Here's the drawing with two shaded views (mm, measured from the low corner). I have some questions. A direction names the side the tool comes from. Give positions to 0.01 mm unless a question says otherwise; leave off trailing zeros. Loops run counter-clockwise (first coordinate to the right, second up) from the corner with the lowest first, then second, coordinate; pieces in that order, holes last. Notation, with made-up numbers: (59, 32.5) - (85, 32.5) arc R8 cw to (85, 43.5) - close; hole circle Ø5 at (72, 58.25). An arc over 180 degrees is marked (long way). Use one line per item in the form item = value.
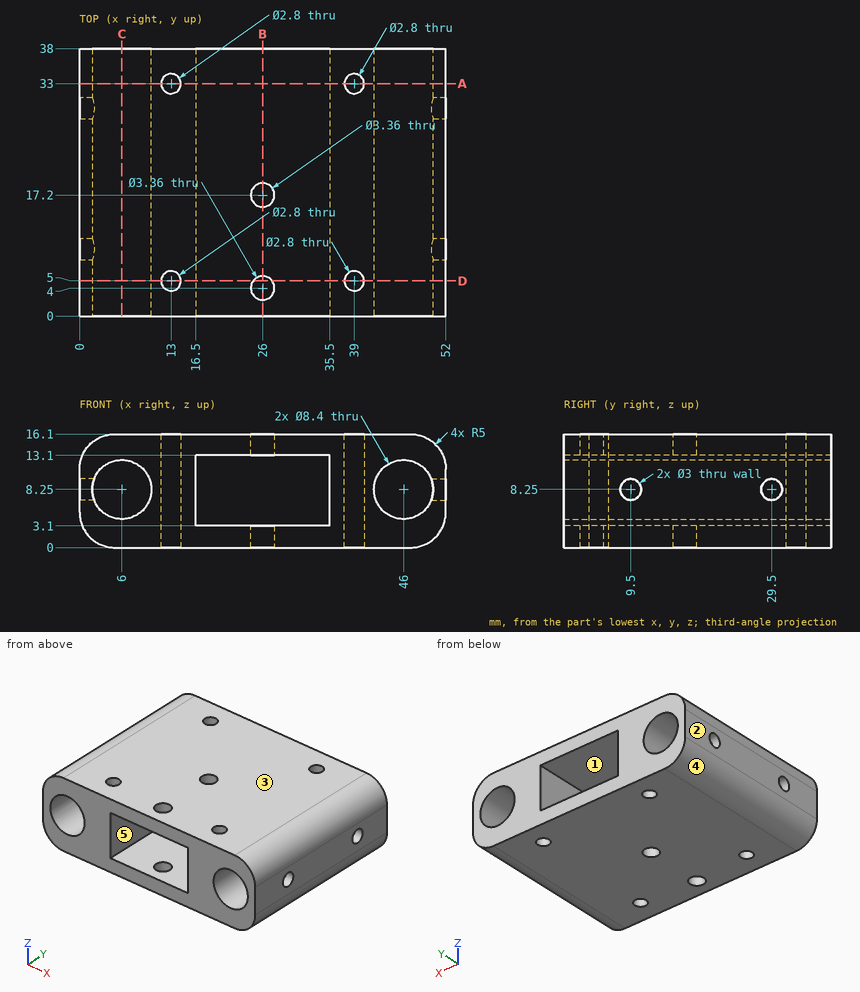
(1) For the marked faces 4 and 5, which set-ups out of +Z, -Z, +X, -X, +Y, -Y let a thin tool reach every point of the face, with its end or its side?
Geometry says:
face_4 = -Z, -X, +Y, -Y
face_5 = +Y, -Y
(2) If we section it at D-D (y = 5): Give the number of separate pieces and of enclosed holes in the cut face, plus the area to 3 significant figures.
Geometry says:
separate_pieces = 4
enclosed_holes = 2
area = 408 mm²
(3) For P1, Ø3.5, axis at y = 29.5, z = 8.25, coming from the -X side; P2, Ø1.8, axis at y = 29.5, z = 8.25, coming from the -X side, each with a flat end and sliding along its axis, tell me the tip position at first contact or that it passes through.
Geometry says:
P1 = 0
P2 = 10.1
(4) Thinking about a two-plate mould opening in X: for the marked faces 1, 2 and 3, which applies, pulls with the +X half, pulls with the -X half, needs draft (parallel to the pull), parting line crosses it, or undercut?
Geometry says:
face_1 = undercut
face_2 = pulls with the -X half
face_3 = needs draft
(5) If I drill on probe 1 along Y at (x, z) = (26, 14.2); probe 2 along Y at (x, z) = (39, 4.75); probe 3 along X at (y, z) = (3, 8.5), over which ranges is the centre line in solid material (lowest first)?
Geometry says:
probe_1 = 0 to 2.32, 5.68 to 15.52, 18.88 to 38
probe_2 = 0 to 3.6, 6.4 to 31.6, 34.4 to 38
probe_3 = 0 to 1.81, 10.19 to 16.5, 35.5 to 41.81, 50.19 to 52
(6) If we section it at B-B (x = 26): List the corners of the cut face in (y, z) for me.
Geometry says:
outline = (0, 0) - (2.32, 0) - (2.32, 3.1) - (0, 3.1) - close; (0, 13.1) - (2.32, 13.1) - (2.32, 16.1) - (0, 16.1) - close; (5.68, 0) - (15.52, 0) - (15.52, 3.1) - (5.68, 3.1) - close; (5.68, 13.1) - (15.52, 13.1) - (15.52, 16.1) - (5.68, 16.1) - close; (18.88, 0) - (38, 0) - (38, 3.1) - (18.88, 3.1) - close; (18.88, 13.1) - (38, 13.1) - (38, 16.1) - (18.88, 16.1) - close
(7) If we section it at A-A (y = 33): List the corners of the cut face in (x, z) for me, plus the area to 3 significant figures.
Geometry says:
outline = (0, 5) arc R5 ccw to (5, 0) - (11.6, 0) - (11.6, 16.1) - (5, 16.1) arc R5 ccw to (0, 11.1) - close; (14.4, 0) - (37.6, 0) - (37.6, 16.1) - (14.4, 16.1) - close; (40.4, 0) - (47, 0) arc R5 ccw to (52, 5) - (52, 11.1) arc R5 ccw to (47, 16.1) - (40.4, 16.1) - close; hole circle Ø8.4 at (6, 8.25); hole (16.5, 3.1) - (35.5, 3.1) - (35.5, 13.1) - (16.5, 13.1) - close; hole circle Ø8.4 at (46, 8.25)
area = 425 mm²
(8) If we section it at C-C (x = 6): List the corners of the cut face in (y, z) for me, plus the area to 3 significant figures.
Geometry says:
outline = (0, 0) - (38, 0) - (38, 4.05) - (0, 4.05) - close; (0, 12.45) - (38, 12.45) - (38, 16.1) - (0, 16.1) - close
area = 293 mm²
